```python
from build123d import *

# Parameters (mm, degrees)
F0_R      = 4.25
F0_R_2    = 20.5
F1_DEPTH  = 6
F3_R      = 7
F3_R_2    = 22.5
F4_DEPTH  = 6
F5_R      = 22.5
F5_R_2    = 20.5
F6_DEPTH  = 112
F9_DEPTH  = 106
F10_DEPTH = 50.8


with BuildPart() as f1:
    # F0 (on Front) → F1 (new body)
    with BuildSketch(Plane.XZ):
        with BuildLine():
            Line((-65.399358, 37.958743), (-74.524437, 9.450272))
            ThreePointArc((-74.524437, 9.450272), (-74.799113, -8.544758), (-65.030261, -23.659853))
            Line((-65.030261, -23.659853), (-42.184567, -43.000853))
            ThreePointArc((-42.184567, -43.000853), (-32.045044, -45.1793), (-24.600642, -37.958743))
            Line((-24.600642, -37.958743), (-15.475563, -9.450272))
            ThreePointArc((-15.475563, -9.450272), (-15.200887, 8.544758), (-24.969739, 23.659853))
            Line((-24.969739, 23.659853), (-47.815433, 43.000853))
            ThreePointArc((-47.815433, 43.000853), (-57.954956, 45.1793), (-65.399358, 37.958743))
        make_face()
        with Locations((-35.077055, -34.605421)):
            Circle(F0_R, mode=Mode.SUBTRACT)
        with Locations((-45, 0)):
            Circle(F0_R_2, mode=Mode.SUBTRACT)
        with Locations((-54.922945, 34.605421)):
            Circle(F0_R, mode=Mode.SUBTRACT)
        with BuildLine():
            ThreePointArc((24.969739, 23.659853), (15.200887, 8.544758), (15.475563, -9.450272))
            Line((15.475563, -9.450272), (24.600642, -37.958743))
            ThreePointArc((24.600642, -37.958743), (32.045044, -45.1793), (42.184567, -43.000853))
            Line((42.184567, -43.000853), (65.030261, -23.659853))
            ThreePointArc((65.030261, -23.659853), (74.799113, -8.544758), (74.524437, 9.450272))
            Line((74.524437, 9.450272), (65.399358, 37.958743))
            ThreePointArc((65.399358, 37.958743), (57.954956, 45.1793), (47.815433, 43.000853))
            Line((47.815433, 43.000853), (24.969739, 23.659853))
        make_face()
        with Locations((35.077055, -34.605421)):
            Circle(F0_R, mode=Mode.SUBTRACT)
        with Locations((45, 0)):
            Circle(F0_R_2, mode=Mode.SUBTRACT)
        with Locations((54.922945, 34.605421)):
            Circle(F0_R, mode=Mode.SUBTRACT)
    extrude(amount=F1_DEPTH)



with BuildPart() as f4:
    # F3 (on offset) → F4 (new body)
    with BuildSketch(Plane.XZ.offset(118)):
        with BuildLine():
            Line((15.254945, -8.731077), (22.125498, -32.137697))
            ThreePointArc((22.125498, -32.137697), (27.239468, -38.087585), (35.084542, -38.180598))
            Line((35.084542, -38.180598), (57.43136, -28.398262))
            ThreePointArc((57.43136, -28.398262), (73.095541, -13.101166), (74.745055, 8.731077))
            Line((74.745055, 8.731077), (67.874502, 32.137697))
            ThreePointArc((67.874502, 32.137697), (62.760532, 38.087585), (54.915458, 38.180598))
            Line((54.915458, 38.180598), (32.56864, 28.398262))
            ThreePointArc((32.56864, 28.398262), (16.904459, 13.101166), (15.254945, -8.731077))
        make_face()
        with Locations((31.264906, -29.455003)):
            Circle(F3_R, mode=Mode.SUBTRACT)
        with Locations((45, 0)):
            Circle(F3_R_2, mode=Mode.SUBTRACT)
        with Locations((58.735094, 29.455003)):
            Circle(F3_R, mode=Mode.SUBTRACT)
        with BuildLine():
            ThreePointArc((-54.915458, 38.180598), (-62.760532, 38.087585), (-67.874502, 32.137697))
            Line((-67.874502, 32.137697), (-74.745055, 8.731077))
            ThreePointArc((-74.745055, 8.731077), (-73.095541, -13.101166), (-57.43136, -28.398262))
            Line((-57.43136, -28.398262), (-35.084542, -38.180598))
            ThreePointArc((-35.084542, -38.180598), (-27.239468, -38.087585), (-22.125498, -32.137697))
            Line((-22.125498, -32.137697), (-15.254945, -8.731077))
            ThreePointArc((-15.254945, -8.731077), (-16.904459, 13.101166), (-32.56864, 28.398262))
            Line((-32.56864, 28.398262), (-54.915458, 38.180598))
        make_face()
        with Locations((-31.264906, -29.455003)):
            Circle(F3_R, mode=Mode.SUBTRACT)
        with Locations((-45, 0)):
            Circle(F3_R_2, mode=Mode.SUBTRACT)
        with Locations((-58.735094, 29.455003)):
            Circle(F3_R, mode=Mode.SUBTRACT)
    extrude(amount=-F4_DEPTH)


with BuildPart() as f6:
    # F5 (on face) → F6 (new body, through all)
    with BuildSketch(Plane.XZ.offset(6)):
        with Locations((-45, 0)):
            Circle(F5_R)
        with Locations((-45, 0)):
            Circle(F5_R_2, mode=Mode.SUBTRACT)
        with Locations((45, 0)):
            Circle(F5_R)
        with Locations((45, 0)):
            Circle(F5_R_2, mode=Mode.SUBTRACT)
    extrude(amount=F6_DEPTH)

    # F7: union F4
    add(f4.part)


with BuildPart() as f1_1:
    add(f1.part)

    add(f6.part)  # F9 merges F6
    # F8 (on face) → F9 (join, through all)
    with BuildSketch(Plane.XZ.offset(6)):
        with BuildLine():
            ThreePointArc((-45, 22.5), (-29.090097, 15.909903), (-22.5, 0))
            Line((-22.5, 0), (22.5, 0))
            ThreePointArc((22.5, 0), (29.090097, 15.909903), (45, 22.5))
            Line((45, 22.5), (-45, 22.5))
        make_face()
    extrude(amount=F9_DEPTH)

    # F9_face (on face) → F10 (join)
    with BuildSketch(Plane(origin=(0, -59, 22.5), x_dir=(1, 0, 0), z_dir=(0, 0, 1))):
        Polygon((45, -53), (45, 53), (23.675132, 53), (-23.675132, 53), (-45, 53), (-45, -53), (-23.675132, -53), (23.675132, -53), align=None)
    extrude(amount=F10_DEPTH)


solid = f1_1.part
```
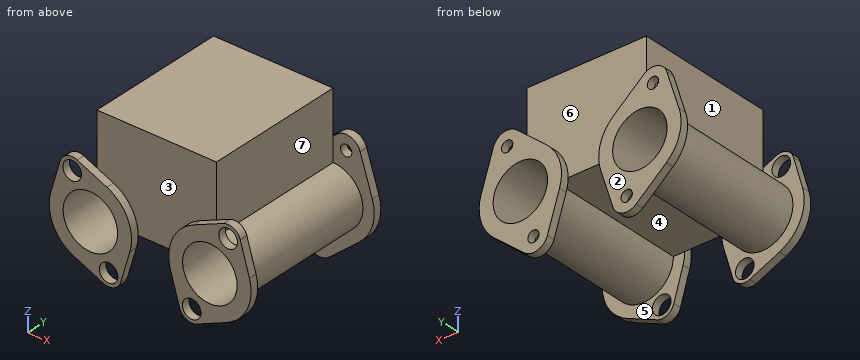
The listing builds one solid part. Answer for the finished solid, in the listing's coordinates (mm). Face numbers are marked on the shaded views. A direction names the side the tool comes from. Coordinates: 2 decimals unless noted, no trailing zeros. Write each loop counter-clockwise with the first axis right and the second up, starting at its lowest first coordinate (ties: lowest second). Pieces come first, ordered by that corner, then holes. Notation, with made-up numbers: (-26, 85) - (-7, 85) arc R6 ccw to (-7, 89) - close; hole circle Ø1 at (53, 65). An arc over 180 degrees is marked (long way). Return JSON: item names as keys, results as strings. Group by question number.
Q1. Which of the six approach directions +Z, -Z, +X, -X, +Y, -Y give full straight-line access (tool end or side, diameter ignored) to the marked faces 4, 5, 6 and 7?
Q2. The part is cut by section B-B on z = -17. State how many separate pieces and enclosed holes the cut face has, and give its area (3 significant figures).
Q3. For a pull along Y with two mould halves and no side action, classify the marked faces 1, 2 and 3 as +Y half, -Y half, draft (parallel to the pull), parting line (faces both ways), or undercut.
Q4. The part is cut by section C-C on x = 63. Write down the section's boundary in (y, z), and give its area (3 significant figures).
Q5. The part is cut by section A-A on y = -49. Write down the section's boundary in (x, z).
Q6. Find the intervals of material crossed by line 1 along Z through (x, y) = (-46, -78.5); line 2 along Y through (x, z) = (48.5, -25.5); line 3 along X through (y, z) = (-16.5, -15), in increasing order. Write a range as [from, to].
Q7. Flat-ended cylindrical pins translate along their axes: pin 1 Ø5 at (x, z) = (-54.92, 34.61) entering from +Y; pin 2 Ø5 at (y, z) = (-53, -19.5) entering from -X; pin 3 Ø10 at (x, z) = (-35.5, 41) entering from +Y. Find the tip coordinate at first contact, or state that the pin passes through.
Q8. The part is cut by section D-D on z = 55. Write down the section's boundary in (x, y).
Evaluation:
{
 "1": {"face 4": "-Z", "face 5": "none", "face 6": "+Z, +Y", "face 7": "+Z, +X"},
 "2": {"separate pieces": "4", "enclosed holes": "0", "area": "2,120 mm2"},
 "3": {"face 1": "undercut", "face 2": "+Y half", "face 3": "-Y half"},
 "4": {"outline": "(-118, -25.24) - (-112, -25.24) - (-112, -13.5) - (-6, -13.5) - (-6, -25.38) - (0, -25.38) - (0, -9.81) - (-118, -9.81) - close; (-118, 9.81) - (0, 9.81) - (0, 42.07) - (-6, 42.07) - (-6, 13.5) - (-112, 13.5) - (-112, 23.9) - (-118, 23.9) - close; (-118, 35.01) - (-112, 35.01) - (-112, 37.97) - (-118, 37.97) - close", "area": "1,260 mm2"},
 "5": {"outline": "(-45, 22.5) arc R22.5 ccw (long way) to (-22.5, 0) - (22.5, 0) arc R22.5 ccw (long way) to (45, 22.5) - (45, 73.3) - (-45, 73.3) - close; hole circle Ø41 at (-45, 0); hole circle Ø41 at (45, 0)"},
 "6": {"line 1": "z = [-22.48, -20.48], [20.48, 22.48]", "line 2": "y = [-118, -112], [-6, 0]", "line 3": "x = [-61.77, -58.97], [-31.03, -28.23], [28.23, 31.03], [58.97, 61.77]"},
 "7": {"pin 1": "stops at y = -112", "pin 2": "stops at x = -59.74", "pin 3": "stops at y = -6"},
 "8": {"outline": "(-45, -112) - (45, -112) - (45, -6) - (-45, -6) - close"}
}
